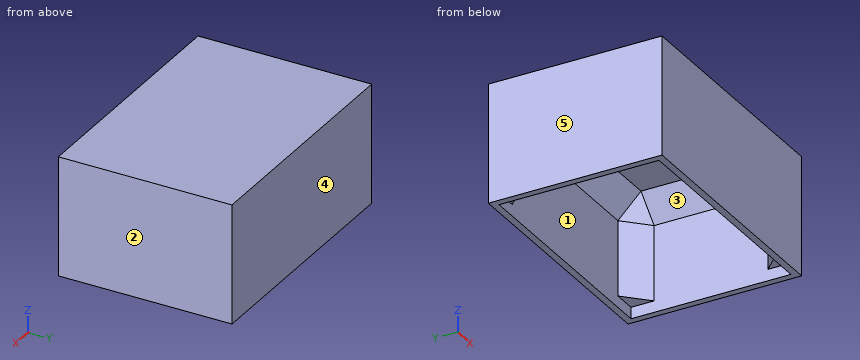
```python
from build123d import *

# Parameters (mm, degrees)
F0_W     = 108
F0_H     = 76
F0_W_2   = 102
F0_H_2   = 70
F1_DEPTH = 47
F2_START = 43
F2_DEPTH = 4
F3_SIZE  = 10.1
F4_DEPTH = 5


with BuildPart() as f1:
    # F0 (on Top) → F1 (new body)
    with BuildSketch(Plane.XY):
        Rectangle(F0_W, F0_H)
        Rectangle(F0_W_2, F0_H_2, mode=Mode.SUBTRACT)
    extrude(amount=F1_DEPTH)

    # F0 (on Top) → F2 (join)
    with BuildSketch(Plane.XY.offset(F2_START)):
        Rectangle(F0_W_2, F0_H_2)
    extrude(amount=F2_DEPTH)

    # F3
    f3_edges = [f1.edges().sort_by_distance(p)[0] for p in [
        (0, 35, 43),
        (-51, 0, 43),
        (0, -35, 43),
        (51, 0, 43),
        (51, 35, 21.5),
        (-51, 35, 21.5),
        (-51, -35, 21.5),
        (51, -35, 21.5),
    ]]
    chamfer(f3_edges, length=F3_SIZE)

    # F0 (on Top) → F4 (join)
    with BuildSketch(Plane.XY):
        Rectangle(F0_W, F0_H)
        Rectangle(F0_W_2, F0_H_2, mode=Mode.SUBTRACT)
    extrude(amount=-F4_DEPTH)


solid = f1.part
```
CAD build for the part. Positions are in the model's coordinates, mm. Face numbers are marked on the shaded views. A direction names the side the tool comes from. Round coordinates to 2 decimals unless told otherwise and drop trailing zeros. Order: outer loops, then holes, each group sorted by start corner. A loop starts at its lowest first (then second) coordinate and runs counter-clockwise, first axis right, second up.
Q1. Slice it at A-A (z = 40.5). Write the cut outline in (x, y), and give its area (3 significant figures).
Q2. Which spindle directions (+Z, -Z, +X, -X, +Y, -Y) get a long thin tool onto all of the face, cutting with end or side? Do the marked faces 1 and 2. Say none if no direction does.
Q3. Drop flat-ended pins along their axis: pin 1 (10 mm diameter, centred on x = 6, y = 18.5, fed in from -Z); pin 2 (8 mm diameter, centred on x = -47.5, y = 30.5, fed in from -Z); pin 3 (3 mm diameter, centred on x = -48.5, y = -31, fed in from -Z). Give the stop position or say it passes through.
Q4. Wall check: L1, parallel to Y at x = -14, z = 22; L2, parallel to X at y = 23.5, z = 17.5; L3, parallel to Z at x = -26, y = 8.5. Give the ranges that are in metal, low to high.
Q5. Slice it at B-B (y = 3). Write the cut outline in (x, z), and give its area (3 significant figures).
Q6. Slice it at D-D (z = 12). Write the cut outline in (x, y), and give its area (3 significant figures).
Q7. Two-plate mould, pull along X, no slides. Class the marked faces 3, 4 and 5: pulls with the +X half, pulls with the -X half, needs draft (parallel to the pull), parting line crosses it, or undercut.
Q8. Slice it at C-C (x = -26.5). Write the cut outline in (y, z).
Results below:
1. outline: (-54, -38) - (54, -38) - (54, 38) - (-54, 38) - close; hole (-43.4, -24.9) - (-40.9, -27.4) - (40.9, -27.4) - (43.4, -24.9) - (43.4, 24.9) - (40.9, 27.4) - (-40.9, 27.4) - (-43.4, 24.9) - close
1. area: 3,460 mm2
2. face 1: -Z
2. face 2: +Z, -Z, +X, +Y, -Y
3. pin 1: stops at z = 43
3. pin 2: stops at z = -5
3. pin 3: stops at z = 0
4. L1: y = -38 to -35, 35 to 38
4. L2: x = -54 to -51, 51 to 54
4. L3: z = 43 to 47
5. outline: (-54, -5) - (-51, -5) - (-51, 32.9) - (-40.9, 43) - (40.9, 43) - (51, 32.9) - (51, -5) - (54, -5) - (54, 47) - (-54, 47) - close
5. area: 822 mm2
6. outline: (-54, -38) - (54, -38) - (54, 38) - (-54, 38) - close; hole (-51, -24.9) - (-40.9, -35) - (40.9, -35) - (51, -24.9) - (51, 24.9) - (40.9, 35) - (-40.9, 35) - (-51, 24.9) - close
6. area: 1,270 mm2
7. face 3: undercut
7. face 4: needs draft
7. face 5: pulls with the -X half
8. outline: (-38, -5) - (-35, -5) - (-35, 32.9) - (-24.9, 43) - (24.9, 43) - (35, 32.9) - (35, -5) - (38, -5) - (38, 47) - (-38, 47) - close
